```python
from build123d import *

# Parameters (mm, degrees)
F0_R     = 38.75
F0_W     = 10
F0_H     = 10
F3_DEPTH = 6
F5_R     = 2.5
F6_DEPTH = 12.5


with BuildPart() as f3:
    # F0 (on Front) → F3 (new body, symmetric)
    with BuildSketch(Plane.XZ):
        Circle(F0_R)
        with BuildLine():
            ThreePointArc((29.5803989155, 5), (29.8949156836, 2.5087878084), (30, 0))
            ThreePointArc((30, 0), (29.8949156836, -2.5087878084), (29.5803989155, -5))
            ThreePointArc((29.5803989155, -5), (21.2132034356, -21.2132034356), (5, -29.5803989155))
            ThreePointArc((5, -29.5803989155), (0, -30), (-5, -29.5803989155))
            ThreePointArc((-5, -29.5803989155), (-21.2132034356, -21.2132034356), (-29.5803989155, -5))
            ThreePointArc((-29.5803989155, -5), (-30, 0), (-29.5803989155, 5))
            ThreePointArc((-29.5803989155, 5), (-21.2132034356, 21.2132034356), (-5, 29.5803989155))
            ThreePointArc((-5, 29.5803989155), (0, 30), (5, 29.5803989155))
            ThreePointArc((5, 29.5803989155), (21.2132034356, 21.2132034356), (29.5803989155, 5))
        make_face(mode=Mode.SUBTRACT)
        with BuildLine():
            Line((5, 5), (5, 29.5803989155))
            ThreePointArc((5, 29.5803989155), (0, 30), (-5, 29.5803989155))
            Line((-5, 29.5803989155), (-5, 5))
            Line((-5, 5), (5, 5))
        make_face()
        with BuildLine():
            ThreePointArc((29.5803989155, -5), (29.8949156836, -2.5087878084), (30, 0))
            ThreePointArc((30, 0), (29.8949156836, 2.5087878084), (29.5803989155, 5))
            Line((29.5803989155, 5), (5, 5))
            Line((5, 5), (5, -5))
            Line((5, -5), (29.5803989155, -5))
        make_face()
        Rectangle(F0_W, F0_H)
        with BuildLine():
            Line((-5, -5), (-5, 5))
            Line((-5, 5), (-29.5803989155, 5))
            ThreePointArc((-29.5803989155, 5), (-30, 0), (-29.5803989155, -5))
            Line((-29.5803989155, -5), (-5, -5))
        make_face()
        with BuildLine():
            ThreePointArc((-5, -29.5803989155), (0, -30), (5, -29.5803989155))
            Line((5, -29.5803989155), (5, -5))
            Line((5, -5), (-5, -5))
            Line((-5, -5), (-5, -29.5803989155))
        make_face()
    extrude(amount=F3_DEPTH, both=True)

    # F1 (on Right) → F4 (revolve, cut)
    with BuildSketch(Plane.YZ):
        with BuildLine():
            Line((3.75, 36), (3.75, 40))
            Line((3.75, 40), (-3.75, 40))
            Line((-3.75, 40), (-3.75, 36))
            ThreePointArc((-3.75, 36), (-2.7248737342, 33.5251262658), (-0.25, 32.5))
            Line((-0.25, 32.5), (0.25, 32.5))
            ThreePointArc((0.25, 32.5), (2.7248737342, 33.5251262658), (3.75, 36))
        make_face()
    revolve(axis=Axis((0, -2.0112972707, 0), (0, -1, 0)), mode=Mode.SUBTRACT)

    # F5 (on Front) → F6 (cut, symmetric)
    with BuildSketch(Plane.XZ):
        Circle(F5_R)
    extrude(amount=F6_DEPTH, both=True, mode=Mode.SUBTRACT)


solid = f3.part
```
Source: CAD feature listing. Evaluate the final solid. Frame: model axes, mm. A direction names the side the tool comes from. Round coordinates to 2 decimals unless told otherwise and drop trailing zeros. Loops run counter-clockwise (first coordinate to the right, second up) from the corner with the lowest first, then second, coordinate; pieces in that order, holes last. Notation, with made-up numbers: M -22.5,55 L 23.5,55 A8 ccw 23.5,65 Z; hole C 32.25,-19.75 d6. An arc over 180 degrees is marked long. Use a Markdown table: item, result. Add a question column.
1. Section query B-B on y = 5. Return the cut outline in (x, z), then the cut area to 3 significant figures.
2. Section query A-A on z = 0. Return the cut outline in (x, y), then the cut area to 3 significant figures.
3. Reachability of faces 4 (the cylindrical face through (-9.76, 0, 31)), 5 (the flat face through (-1, 6, -8)), 6 (the flat face through (-5, 0, -17)) from +Z, -Z, +X, -X, +Y, -Y: full face, straight path, thin tool, end or side. Return the list, or none.
4. Section query D-D on x = -26.5. Give the number of separate pieces and of enclosed holes in the cut face, then the cut area to 3 significant figures.
5. Contact query for flat-ended pins moving along their axis: P1, Ø3.5, axis at y = 2.5, z = -11.5, coming from the -X side; P2, Ø6, axis at x = -29.5, y = -3.5, coming from the -Z side; P3, Ø5, axis at y = 0, z = 7.5, coming from the -X side. Output: stop coordinate, or through.
6. Mould query, pull axis X, two halves, no side actions, for faces 1 (the cylindrical face through (-8.4, 4.86, -37.83)), 2 (the cylindrical face through (21.029, -0.084, 21.396)), 3 (the flat face through (26, -3.75, 26)). Classes: pulls with the +X half, pulls with the -X half, needs draft (parallel to the pull), parting line crosses it, or undercut.
7. Line query: line 1 (Y direction, x = -27, z = 25); line 2 (Z direction, x = 0, y = 0.5); line 3 (X direction, y = -4, z = -17.5). Output: solid intervals per line, ascending.
8. Section query C-C on x = 0. Return the cut outline in (y, z), then the cut area to 3 significant figures.
Reported:
| question | item | result |
|---|---|---|
| 1 | outline | C 0,0 d77.5; hole M -29.58,-5 A30 ccw -5,-29.58 L -5,-5 Z; hole M -29.58,5 L -5,5 L -5,29.58 A30 ccw Z; hole C 0,0 d5; hole M 5,-29.58 A30 ccw 29.58,-5 L 5,-5 Z; hole M 5,5 L 29.58,5 A30 ccw 5,29.58 Z |
| 1 | area | 2,960 mm² |
| 2 | outline | M -38.75,-6 L -2.5,-6 L -2.5,6 L -38.75,6 L -38.75,3.75 L -36,3.75 A3.5 cw -32.5,0.25 L -32.5,-0.25 A3.5 cw -36,-3.75 L -38.75,-3.75 Z; M 2.5,-6 L 38.75,-6 L 38.75,-3.75 L 36,-3.75 A3.5 cw 32.5,-0.25 L 32.5,0.25 A3.5 cw 36,3.75 L 38.75,3.75 L 38.75,6 L 2.5,6 Z |
| 2 | area | 787 mm² |
| 3 | face 4 | none |
| 3 | face 5 | +Z, -Z, +X, -X, +Y |
| 3 | face 6 | +Y, -Y |
| 4 | separate pieces | 3 |
| 4 | enclosed holes | 0 |
| 4 | area | 337 mm² |
| 5 | P1 | stops at x = -37.36 |
| 5 | P2 | stops at z = -28.26 |
| 5 | P3 | stops at x = -32.54 |
| 6 | face 1 | parting line crosses it |
| 6 | face 2 | undercut |
| 6 | face 3 | needs draft |
| 7 | line 1 | y = -6 to -3.75, 3.75 to 6 |
| 7 | line 2 | z = -32.51 to -2.5, 2.5 to 32.51 |
| 7 | line 3 | x = -34.57 to -24.37, -5 to 5, 24.37 to 34.57 |
| 8 | outline | M -6,-38.75 L -3.75,-38.75 L -3.75,-36 A3.5 cw -0.25,-32.5 L 0.25,-32.5 A3.5 cw 3.75,-36 L 3.75,-38.75 L 6,-38.75 L 6,-2.5 L -6,-2.5 Z; M -6,2.5 L 6,2.5 L 6,38.75 L 3.75,38.75 L 3.75,36 A3.5 cw 0.25,32.5 L -0.25,32.5 A3.5 cw -3.75,36 L -3.75,38.75 L -6,38.75 Z |
| 8 | area | 787 mm² |
